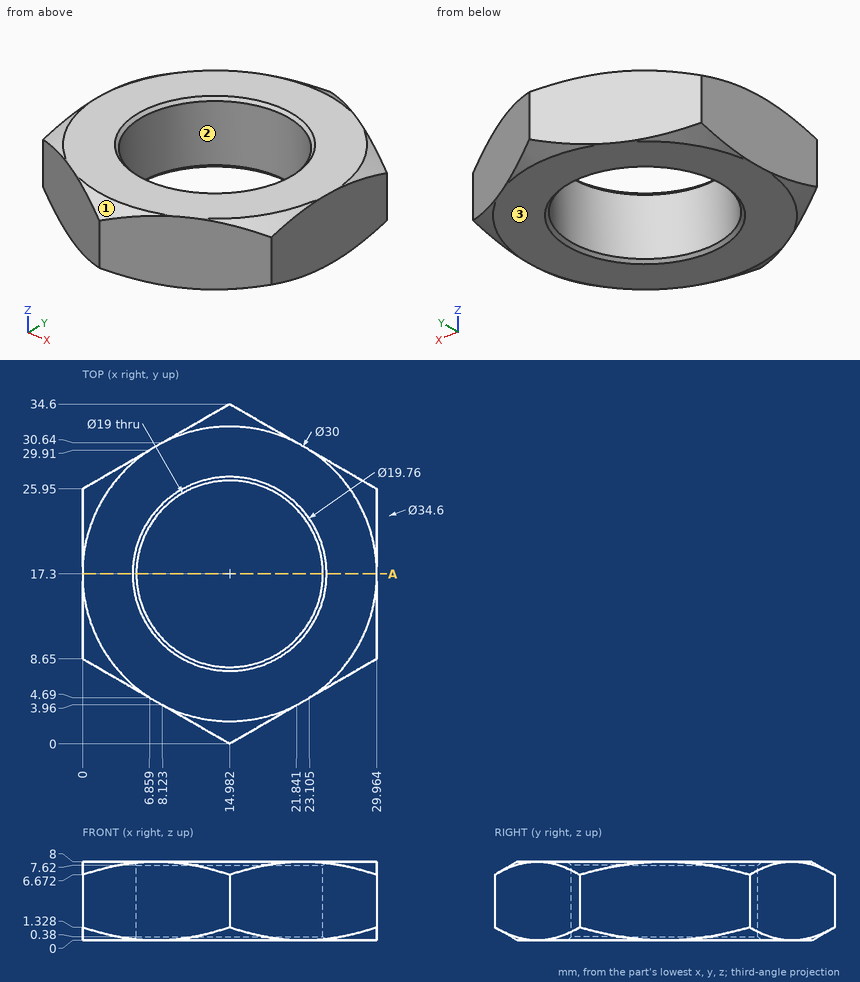
Design review of the part shown in the three views and the two pictorial views. Dimensions are in mm from the part's minimum x, y and z. Coordinates: 2 decimals unless noted, no trailing zeros. Write each loop counter-clockwise with the first axis right and the second up, starting at its lowest first coordinate (ties: lowest second). Pieces come first, ordered by that corner, then holes. Notation, with made-up numbers: (61, 8.5) - (103, 8.5) arc R22 cw to (103, 39.5) - close; hole circle Ø3 at (-3.75, 65). An arc over 180 degrees is marked (long way). Write item = value, one per line.
(1) For P1, Ø4, axis at x = 21, z = 2, coming from the +Y side; P2, Ø1.5, axis at x = 6.5, z = 2.5, coming from the -Y side (1 decimal), all flat-tipped, find the tip position at first contact; note any pin that passes through.
Result sheet:
P1 = 32.28
P2 = 4.5
(2) For line 1 (Y direction, x = 22.25, z = 2) (1 decimal); line 2 (X direction, y = 18, z = 7) (1 decimal); line 3 (Y direction, x = 22.5, z = 6.75) (1 decimal), list the stretches that pass through material, from the lowest coordinate up. Write a range as [from, to].
Result sheet:
line_1 = [4.2, 11.2], [23.4, 30.4]
line_2 = [0, 5.5], [24.5, 30]
line_3 = [4.3, 11.5], [23.1, 30.3]
(3) Mouldability with a two-part tool opening along X and no side actions: class the marked faces 1, 2 and 3 as pulls with the +X half, pulls with the -X half, needs draft (parallel to the pull), parting line crosses it, or undercut.
Result sheet:
face_1 = parting line crosses it
face_2 = undercut
face_3 = needs draft
(4) Consider section A-A, the plane y = 17.3. Give the boundary of the cut face in (x, z) (1 decimal).
Result sheet:
outline = (0, 0) - (5.1, 0) - (5.5, 0.4) - (5.5, 7.6) - (5.1, 8) - (0, 8) - close; (24.5, 0.4) - (24.9, 0) - (30, 0) - (30, 8) - (24.9, 8) - (24.5, 7.6) - close
